For this review, take the finished solid that the model builds, in its own axes (mm). Face numbers are marked on the shaded views. A direction names the side the tool comes from. Coordinates: 2 decimals unless noted, no trailing zeros. Write each loop counter-clockwise with the first axis right and the second up, starting at its lowest first coordinate (ties: lowest second). Pieces come first, ordered by that corner, then holes.
```python
from build123d import *

# Parameters (mm, degrees)
F1_DEPTH = 2
F2_R     = 1
F3_DEPTH = 2.001


with BuildPart() as f1:
    # F0 (on Top) → F1 (new body)
    with BuildSketch(Plane.XY):
        with BuildLine():
            ThreePointArc((7.437103, -0.969279), (7.484259, -0.485659), (7.5, 0))
            ThreePointArc((7.5, 0), (7.484259, 0.485659), (7.437103, 0.969279))
            ThreePointArc((7.437103, 0.969279), (7.35589, 1.463177), (7.241914, 1.950559))
            ThreePointArc((7.241914, 1.950559), (6.929096, 2.870126), (6.50006, 3.741553))
            ThreePointArc((6.50006, 3.741553), (6.236022, 4.166777), (5.94421, 4.573442))
            ThreePointArc((5.94421, 4.573442), (5.303301, 5.303301), (4.573442, 5.94421))
            ThreePointArc((4.573442, 5.94421), (4.166777, 6.236022), (3.741553, 6.50006))
            ThreePointArc((3.741553, 6.50006), (2.870126, 6.929096), (1.950559, 7.241914))
            ThreePointArc((1.950559, 7.241914), (1.463177, 7.35589), (0.969279, 7.437103))
            ThreePointArc((0.969279, 7.437103), (0, 7.5), (-0.969279, 7.437103))
            ThreePointArc((-0.969279, 7.437103), (-1.463177, 7.35589), (-1.950559, 7.241914))
            ThreePointArc((-1.950559, 7.241914), (-2.870126, 6.929096), (-3.741553, 6.50006))
            ThreePointArc((-3.741553, 6.50006), (-4.166777, 6.236022), (-4.573442, 5.94421))
            ThreePointArc((-4.573442, 5.94421), (-5.303301, 5.303301), (-5.94421, 4.573442))
            ThreePointArc((-5.94421, 4.573442), (-6.236022, 4.166777), (-6.50006, 3.741553))
            ThreePointArc((-6.50006, 3.741553), (-6.929096, 2.870126), (-7.241914, 1.950559))
            ThreePointArc((-7.241914, 1.950559), (-7.35589, 1.463177), (-7.437103, 0.969279))
            ThreePointArc((-7.437103, 0.969279), (-7.5, 0), (-7.437103, -0.969279))
            ThreePointArc((-7.437103, -0.969279), (-7.35589, -1.463177), (-7.241914, -1.950559))
            ThreePointArc((-7.241914, -1.950559), (-6.929096, -2.870126), (-6.50006, -3.741553))
            ThreePointArc((-6.50006, -3.741553), (-6.236022, -4.166777), (-5.94421, -4.573442))
            ThreePointArc((-5.94421, -4.573442), (-5.303301, -5.303301), (-4.573442, -5.94421))
            ThreePointArc((-4.573442, -5.94421), (-4.166777, -6.236022), (-3.741553, -6.50006))
            ThreePointArc((-3.741553, -6.50006), (-2.870126, -6.929096), (-1.950559, -7.241914))
            ThreePointArc((-1.950559, -7.241914), (-1.463177, -7.35589), (-0.969279, -7.437103))
            ThreePointArc((-0.969279, -7.437103), (0, -7.5), (0.969279, -7.437103))
            ThreePointArc((0.969279, -7.437103), (1.463177, -7.35589), (1.950559, -7.241914))
            ThreePointArc((1.950559, -7.241914), (2.870126, -6.929096), (3.741553, -6.50006))
            ThreePointArc((3.741553, -6.50006), (4.166777, -6.236022), (4.573442, -5.94421))
            ThreePointArc((4.573442, -5.94421), (5.303301, -5.303301), (5.94421, -4.573442))
            ThreePointArc((5.94421, -4.573442), (6.236022, -4.166777), (6.50006, -3.741553))
            ThreePointArc((6.50006, -3.741553), (6.929096, -2.870126), (7.241914, -1.950559))
            ThreePointArc((7.241914, -1.950559), (7.35589, -1.463177), (7.437103, -0.969279))
        make_face()
        with BuildLine():
            ThreePointArc((7.437103, 0.969279), (7.484259, 0.485659), (7.5, 0))
            ThreePointArc((7.5, 0), (7.484259, -0.485659), (7.437103, -0.969279))
            Line((7.437103, -0.969279), (9.513775, -0.75))
            Line((9.513775, -0.75), (9.500322, 0))
            Line((9.500322, 0), (9.513775, 0.75))
            Line((9.513775, 0.75), (7.437103, 0.969279))
        make_face()
        with BuildLine():
            ThreePointArc((6.50006, 3.741553), (6.929096, 2.870126), (7.241914, 1.950559))
            Line((7.241914, 1.950559), (9.076594, 2.947854))
            Line((9.076594, 2.947854), (8.777153, 3.635616))
            Line((8.777153, 3.635616), (8.502569, 4.333674))
            Line((8.502569, 4.333674), (6.50006, 3.741553))
        make_face()
        with BuildLine():
            Line((9.076594, -2.947854), (7.241914, -1.950559))
            ThreePointArc((7.241914, -1.950559), (6.929096, -2.870126), (6.50006, -3.741553))
            Line((6.50006, -3.741553), (8.502569, -4.333674))
            Line((8.502569, -4.333674), (8.777153, -3.635616))
            Line((8.777153, -3.635616), (9.076594, -2.947854))
        make_face()
        with BuildLine():
            ThreePointArc((4.573442, 5.94421), (5.303301, 5.303301), (5.94421, 4.573442))
            Line((5.94421, 4.573442), (7.257585, 6.196924))
            Line((7.257585, 6.196924), (6.717742, 6.717742))
            Line((6.717742, 6.717742), (6.196924, 7.257585))
            Line((6.196924, 7.257585), (4.573442, 5.94421))
        make_face()
        with BuildLine():
            Line((7.257585, -6.196924), (5.94421, -4.573442))
            ThreePointArc((5.94421, -4.573442), (5.303301, -5.303301), (4.573442, -5.94421))
            Line((4.573442, -5.94421), (6.196924, -7.257585))
            Line((6.196924, -7.257585), (6.717742, -6.717742))
            Line((6.717742, -6.717742), (7.257585, -6.196924))
        make_face()
        with BuildLine():
            ThreePointArc((1.950559, 7.241914), (2.870126, 6.929096), (3.741553, 6.50006))
            Line((3.741553, 6.50006), (4.333674, 8.502569))
            Line((4.333674, 8.502569), (3.635616, 8.777153))
            Line((3.635616, 8.777153), (2.947854, 9.076594))
            Line((2.947854, 9.076594), (1.950559, 7.241914))
        make_face()
        with BuildLine():
            Line((4.333674, -8.502569), (3.741553, -6.50006))
            ThreePointArc((3.741553, -6.50006), (2.870126, -6.929096), (1.950559, -7.241914))
            Line((1.950559, -7.241914), (2.947854, -9.076594))
            Line((2.947854, -9.076594), (3.635616, -8.777153))
            Line((3.635616, -8.777153), (4.333674, -8.502569))
        make_face()
        with BuildLine():
            ThreePointArc((-0.969279, 7.437103), (0, 7.5), (0.969279, 7.437103))
            Line((0.969279, 7.437103), (0.75, 9.513775))
            Line((0.75, 9.513775), (0, 9.500322))
            Line((0, 9.500322), (-0.75, 9.513775))
            Line((-0.75, 9.513775), (-0.969279, 7.437103))
        make_face()
        with BuildLine():
            Line((0.75, -9.513775), (0.969279, -7.437103))
            ThreePointArc((0.969279, -7.437103), (0, -7.5), (-0.969279, -7.437103))
            Line((-0.969279, -7.437103), (-0.75, -9.513775))
            Line((-0.75, -9.513775), (0, -9.500322))
            Line((0, -9.500322), (0.75, -9.513775))
        make_face()
        with BuildLine():
            ThreePointArc((-3.741553, 6.50006), (-2.870126, 6.929096), (-1.950559, 7.241914))
            Line((-1.950559, 7.241914), (-2.947854, 9.076594))
            Line((-2.947854, 9.076594), (-3.635616, 8.777153))
            Line((-3.635616, 8.777153), (-4.333674, 8.502569))
            Line((-4.333674, 8.502569), (-3.741553, 6.50006))
        make_face()
        with BuildLine():
            Line((-2.947854, -9.076594), (-1.950559, -7.241914))
            ThreePointArc((-1.950559, -7.241914), (-2.870126, -6.929096), (-3.741553, -6.50006))
            Line((-3.741553, -6.50006), (-4.333674, -8.502569))
            Line((-4.333674, -8.502569), (-3.635616, -8.777153))
            Line((-3.635616, -8.777153), (-2.947854, -9.076594))
        make_face()
        with BuildLine():
            ThreePointArc((-5.94421, 4.573442), (-5.303301, 5.303301), (-4.573442, 5.94421))
            Line((-4.573442, 5.94421), (-6.196924, 7.257585))
            Line((-6.196924, 7.257585), (-6.717742, 6.717742))
            Line((-6.717742, 6.717742), (-7.257585, 6.196924))
            Line((-7.257585, 6.196924), (-5.94421, 4.573442))
        make_face()
        with BuildLine():
            Line((-6.196924, -7.257585), (-4.573442, -5.94421))
            ThreePointArc((-4.573442, -5.94421), (-5.303301, -5.303301), (-5.94421, -4.573442))
            Line((-5.94421, -4.573442), (-7.257585, -6.196924))
            Line((-7.257585, -6.196924), (-6.717742, -6.717742))
            Line((-6.717742, -6.717742), (-6.196924, -7.257585))
        make_face()
        with BuildLine():
            ThreePointArc((-7.241914, 1.950559), (-6.929096, 2.870126), (-6.50006, 3.741553))
            Line((-6.50006, 3.741553), (-8.502569, 4.333674))
            Line((-8.502569, 4.333674), (-8.777153, 3.635616))
            Line((-8.777153, 3.635616), (-9.076594, 2.947854))
            Line((-9.076594, 2.947854), (-7.241914, 1.950559))
        make_face()
        with BuildLine():
            Line((-8.502569, -4.333674), (-6.50006, -3.741553))
            ThreePointArc((-6.50006, -3.741553), (-6.929096, -2.870126), (-7.241914, -1.950559))
            Line((-7.241914, -1.950559), (-9.076594, -2.947854))
            Line((-9.076594, -2.947854), (-8.777153, -3.635616))
            Line((-8.777153, -3.635616), (-8.502569, -4.333674))
        make_face()
        with BuildLine():
            ThreePointArc((-7.437103, -0.969279), (-7.5, 0), (-7.437103, 0.969279))
            Line((-7.437103, 0.969279), (-9.513775, 0.75))
            Line((-9.513775, 0.75), (-9.500322, 0))
            Line((-9.500322, 0), (-9.513775, -0.75))
            Line((-9.513775, -0.75), (-7.437103, -0.969279))
        make_face()
    extrude(amount=F1_DEPTH)

    # F2 (on face) → F3 (cut, through all)
    with BuildSketch(Plane.XY.offset(2)):
        Circle(F2_R)
    extrude(amount=-F3_DEPTH, mode=Mode.SUBTRACT)


solid = f1.part
```
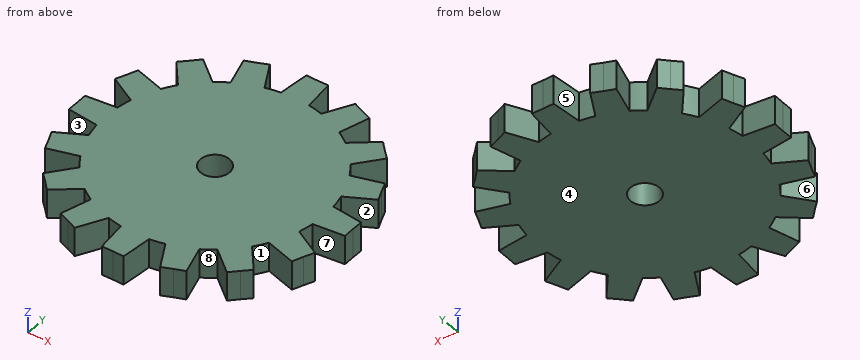
Q1. For probe 1 along X at (y, z) = (7, 1.6); probe 2 along Y at (x, z) = (-7.75, 0.2); probe 3 along Y at (x, z) = (-7.5, 1.65), list the stretches that pass through material, from the lowest coordinate up.
Ans:
probe 1: x = -6.45 to -5.88, -3.89 to 3.89, 5.88 to 6.45
probe 2: y = -4.11 to -2.23, -0.94 to 0.94, 2.23 to 4.11
probe 3: y = -4.04 to -2.09, -0.96 to 0.96, 2.09 to 4.04
Q2. Add section A-A (y = -0.25). State the section outline as (x, z) points, then the cut area to 3 significant figures.
Ans:
outline: (-9.5, 0) - (-0.97, 0) - (-0.97, 2) - (-9.5, 2) - close; (0.97, 0) - (9.5, 0) - (9.5, 2) - (0.97, 2) - close
area: 34.1 mm2
Q3. Draft analysis for pull direction X (two halves, no side actions). For the marked faces 1, 2, 3 and 4, state which applies: +X half, -X half, draft (parallel to the pull), parting line (faces both ways), or undercut.
Ans:
face 1: undercut
face 2: +X half
face 3: -X half
face 4: draft
Q4. Add section B-B (x = 4). State the section outline as (y, z) points.
Ans:
outline: (-8.63, 0) - (-7.37, 0) - (-7.37, 2) - (-8.63, 2) - close; (-6.34, 0) - (6.34, 0) - (6.34, 2) - (-6.34, 2) - close; (7.37, 0) - (8.63, 0) - (8.63, 2) - (7.37, 2) - close
Q5. Tool access review of the marked faces 5, 6, 7 and 8: name each direction out of +Z, -Z, +X, -X, +Y, -Y from which nothing blocks a thin tool from reaching the whole face with its end or side.
Ans:
face 5: +Z, -Z, +Y
face 6: +Z, -Z, -X
face 7: +Z, -Z, +X
face 8: +Z, -Z
